Build history of the part. All positions in model axes, mm. Face numbers are marked on the shaded views. A direction names the side the tool comes from. Give positions to 0.01 mm unless a question says otherwise; leave off trailing zeros. Order: outer loops, then holes, each group sorted by start corner. A loop starts at its lowest first (then second) coordinate and runs counter-clockwise, first axis right, second up. Notation, with made-up numbers: (78, -40) - (134, -40) arc R25 ccw to (134, -1) - close; hole circle Ø6 at (12, -29.75). An arc over 180 degrees is marked (long way). Write each question's results on one line, items separated by ' | '. Start each with the question number.
1) Cut at C-C on z = 7.25. State how many separate pieces and enclosed holes the cut face has, plus the area to 3 significant figures.
2) Two-plate mould, pull along X, no slides. Class the marked faces 1, 2 and 3: +X half, -X half, draft (parallel to the pull), parting line (faces both ways), or undercut.
3) Cut at B-B on x = 24. List the corners of the cut face in (y, z), plus the area to 3 significant figures.
4) Drill centre lines: line 1 along Y through (x, z) = (0, 6); line 2 along Y through (x, z) = (13.5, 1.5) (3 decimals); line 3 along X through (y, z) = (-15, 6.5). Where is each one in solid material? Low to high. Write a range as from..to.
5) Cut at A-A on y = 0. List the corners of the cut face in (x, z), plus the area to 3 significant figures.
6) Cut at D-D on y = 14.3. List the corners of the cut face in (x, z), plus the area to 3 significant figures.
7) Drop flat-ended pins along their axis: pin 1 Ø7 at (x, y) = (36, 0) entering from -Z; pin 2 Ø2.5 at (x, y) = (-2, -27) entering from +Z; pin 3 Ø1 at (x, z) = (-25, 4) entering from +Y. Give the stop position or say it passes through.
8) Tool access for the marked faces 4, 5 and 6: list every direction of +Z, -Z, +X, -X, +Y, -Y with a clear straight run to the whole face (end or side of a thin tool).
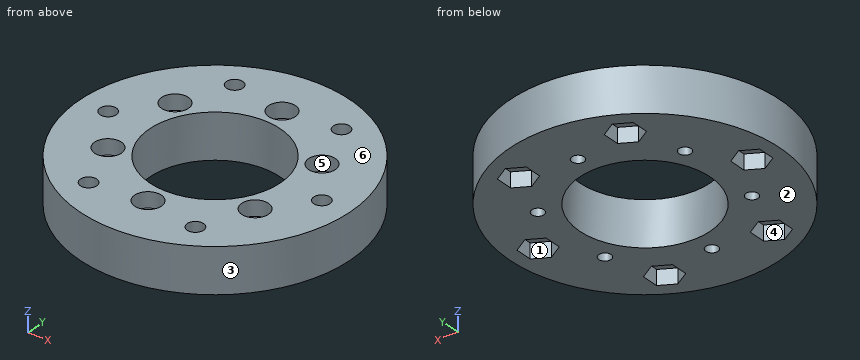
from build123d import *

# Parameters (mm, degrees)
F0_R     = 45.5
F0_R_2   = 2.05
F0_R_3   = 22
F0_R_4   = 2.75
F1_DEPTH = 15
F2_R     = 4.5
F2_R_2   = 2.05
F3_DEPTH = 5.1
F4_DEPTH = 5


with BuildPart() as f1:
    # F0 (on Top) → F1 (new body)
    with BuildSketch(Plane.XY):
        Circle(F0_R)
        Polygon((-22.893044, -28.351915), (-18, -25.526915), (-13.106956, -28.351915), (-13.106956, -34.001915), (-18, -36.826915), (-22.893044, -34.001915), align=None, mode=Mode.SUBTRACT)
        with Locations((-24.768327, -14.3)):
            Circle(F0_R_2, mode=Mode.SUBTRACT)
        with Locations((0, -28.6)):
            Circle(F0_R_2, mode=Mode.SUBTRACT)
        Polygon((13.106956, -34.001915), (13.106956, -28.351915), (18, -25.526915), (22.893044, -28.351915), (22.893044, -34.001915), (18, -36.826915), align=None, mode=Mode.SUBTRACT)
        with Locations((24.768327, -14.3)):
            Circle(F0_R_2, mode=Mode.SUBTRACT)
        Polygon((-36, 5.65), (-31.106956, 2.825), (-31.106956, -2.825), (-36, -5.65), (-40.893044, -2.825), (-40.893044, 2.825), align=None, mode=Mode.SUBTRACT)
        with Locations((-24.768327, 14.3)):
            Circle(F0_R_2, mode=Mode.SUBTRACT)
        Polygon((-13.106956, 34.001915), (-13.106956, 28.351915), (-18, 25.526915), (-22.893044, 28.351915), (-22.893044, 34.001915), (-18, 36.826915), align=None, mode=Mode.SUBTRACT)
        Circle(F0_R_3, mode=Mode.SUBTRACT)
        Polygon((36, -5.65), (31.106956, -2.825), (31.106956, 2.825), (36, 5.65), (40.893044, 2.825), (40.893044, -2.825), align=None, mode=Mode.SUBTRACT)
        with Locations((24.768327, 14.3)):
            Circle(F0_R_2, mode=Mode.SUBTRACT)
        with Locations((0, 28.6)):
            Circle(F0_R_2, mode=Mode.SUBTRACT)
        Polygon((22.893044, 28.351915), (18, 25.526915), (13.106956, 28.351915), (13.106956, 34.001915), (18, 36.826915), (22.893044, 34.001915), align=None, mode=Mode.SUBTRACT)
        Polygon((-31.106956, -2.825), (-31.106956, 2.825), (-36, 5.65), (-40.893044, 2.825), (-40.893044, -2.825), (-36, -5.65), align=None)
        with Locations((-36, 0)):
            Circle(F0_R_4, mode=Mode.SUBTRACT)
        Polygon((-13.106956, -28.351915), (-18, -25.526915), (-22.893044, -28.351915), (-22.893044, -34.001915), (-18, -36.826915), (-13.106956, -34.001915), align=None)
        with Locations((-18, -31.176915)):
            Circle(F0_R_4, mode=Mode.SUBTRACT)
        Polygon((18, -25.526915), (13.106956, -28.351915), (13.106956, -34.001915), (18, -36.826915), (22.893044, -34.001915), (22.893044, -28.351915), align=None)
        with Locations((18, -31.176915)):
            Circle(F0_R_4, mode=Mode.SUBTRACT)
        Polygon((31.106956, 2.825), (31.106956, -2.825), (36, -5.65), (40.893044, -2.825), (40.893044, 2.825), (36, 5.65), align=None)
        with Locations((36, 0)):
            Circle(F0_R_4, mode=Mode.SUBTRACT)
        Polygon((13.106956, 28.351915), (18, 25.526915), (22.893044, 28.351915), (22.893044, 34.001915), (18, 36.826915), (13.106956, 34.001915), align=None)
        with Locations((18, 31.176915)):
            Circle(F0_R_4, mode=Mode.SUBTRACT)
        Polygon((-18, 25.526915), (-13.106956, 28.351915), (-13.106956, 34.001915), (-18, 36.826915), (-22.893044, 34.001915), (-22.893044, 28.351915), align=None)
        with Locations((-18, 31.176915)):
            Circle(F0_R_4, mode=Mode.SUBTRACT)
    extrude(amount=F1_DEPTH)

    # F2 (on face) → F3 (cut)
    with BuildSketch(Plane.XY.offset(15)):
        with Locations((24.768327, 14.3)):
            Circle(F2_R)
        with Locations((24.768327, 14.3)):
            Circle(F2_R_2, mode=Mode.SUBTRACT)
        with Locations((-24.768327, 14.3)):
            Circle(F2_R)
        with Locations((-24.768327, 14.3)):
            Circle(F2_R_2, mode=Mode.SUBTRACT)
        with Locations((0, 28.6)):
            Circle(F2_R)
        with Locations((0, 28.6)):
            Circle(F2_R_2, mode=Mode.SUBTRACT)
        with Locations((-24.768327, -14.3)):
            Circle(F2_R)
        with Locations((-24.768327, -14.3)):
            Circle(F2_R_2, mode=Mode.SUBTRACT)
        with Locations((0, -28.6)):
            Circle(F2_R)
        with Locations((0, -28.6)):
            Circle(F2_R_2, mode=Mode.SUBTRACT)
        with Locations((24.768327, -14.3)):
            Circle(F2_R)
        with Locations((24.768327, -14.3)):
            Circle(F2_R_2, mode=Mode.SUBTRACT)
    extrude(amount=-F3_DEPTH, mode=Mode.SUBTRACT)

    # F0 (on Top) → F4 (cut)
    with BuildSketch(Plane.XY):
        Polygon((-13.106956, -28.351915), (-18, -25.526915), (-22.893044, -28.351915), (-22.893044, -34.001915), (-18, -36.826915), (-13.106956, -34.001915), align=None)
        with Locations((-18, -31.176915)):
            Circle(F0_R_4, mode=Mode.SUBTRACT)
        Polygon((18, -25.526915), (13.106956, -28.351915), (13.106956, -34.001915), (18, -36.826915), (22.893044, -34.001915), (22.893044, -28.351915), align=None)
        with Locations((18, -31.176915)):
            Circle(F0_R_4, mode=Mode.SUBTRACT)
        Polygon((31.106956, 2.825), (31.106956, -2.825), (36, -5.65), (40.893044, -2.825), (40.893044, 2.825), (36, 5.65), align=None)
        with Locations((36, 0)):
            Circle(F0_R_4, mode=Mode.SUBTRACT)
        Polygon((13.106956, 28.351915), (18, 25.526915), (22.893044, 28.351915), (22.893044, 34.001915), (18, 36.826915), (13.106956, 34.001915), align=None)
        with Locations((18, 31.176915)):
            Circle(F0_R_4, mode=Mode.SUBTRACT)
        Polygon((-18, 25.526915), (-13.106956, 28.351915), (-13.106956, 34.001915), (-18, 36.826915), (-22.893044, 34.001915), (-22.893044, 28.351915), align=None)
        with Locations((-18, 31.176915)):
            Circle(F0_R_4, mode=Mode.SUBTRACT)
        Polygon((-31.106956, -2.825), (-31.106956, 2.825), (-36, 5.65), (-40.893044, 2.825), (-40.893044, -2.825), (-36, -5.65), align=None)
        with Locations((-36, 0)):
            Circle(F0_R_4, mode=Mode.SUBTRACT)
    extrude(amount=F4_DEPTH, mode=Mode.SUBTRACT)


solid = f1.part
Results:
1) separate pieces: 1 | enclosed holes: 13 | area: 4,760 mm^2
2) face 1: undercut | face 2: draft | face 3: parting line
3) outline: (-38.66, 0) - (-16.2, 0) - (-16.2, 9.9) - (-18.73, 9.9) - (-18.73, 15) - (-38.66, 15) - close; (-12.4, 0) - (12.4, 0) - (12.4, 9.9) - (9.87, 9.9) - (9.87, 15) - (-9.87, 15) - (-9.87, 9.9) - (-12.4, 9.9) - close; (16.2, 0) - (38.66, 0) - (38.66, 15) - (18.73, 15) - (18.73, 9.9) - (16.2, 9.9) - close | area: 994 mm^2
4) line 1: -45.5..-30.65, -26.55..-22, 22..26.55, 30.65..45.5 | line 2: -43.451..-34.229, -28.125..-17.371, 17.371..28.125, 34.229..43.451 | line 3: -42.96..-26.7, -22.84..-16.09, 16.09..22.84, 26.7..42.96
5) outline: (-45.5, 0) - (-40.89, 0) - (-40.89, 5) - (-38.75, 5) - (-38.75, 15) - (-45.5, 15) - close; (-33.25, 5) - (-31.11, 5) - (-31.11, 0) - (-22, 0) - (-22, 15) - (-33.25, 15) - close; (22, 0) - (31.11, 0) - (31.11, 5) - (33.25, 5) - (33.25, 15) - (22, 15) - close; (38.75, 5) - (40.89, 5) - (40.89, 0) - (45.5, 0) - (45.5, 15) - (38.75, 15) - close | area: 497 mm^2
6) outline: (-43.19, 0) - (-26.82, 0) - (-26.82, 9.9) - (-29.27, 9.9) - (-29.27, 15) - (-43.19, 15) - close; (-22.72, 0) - (-16.72, 0) - (-16.72, 15) - (-20.27, 15) - (-20.27, 9.9) - (-22.72, 9.9) - close; (16.72, 0) - (22.72, 0) - (22.72, 9.9) - (20.27, 9.9) - (20.27, 15) - (16.72, 15) - close; (26.82, 0) - (43.19, 0) - (43.19, 15) - (29.27, 15) - (29.27, 9.9) - (26.82, 9.9) - close | area: 621 mm^2
7) pin 1: z = 5 | pin 2: z = 9.9 | pin 3: y = 38.34
8) face 4: -Z | face 5: +Z | face 6: +Z, +X, -X, +Y, -Y
